```python
from build123d import *

# Parameters (mm, degrees)
BOSS_EXTRU_1_DEPTH = 8
CHANFREIN1_SIZE    = 3


with BuildPart() as part:
    # Esquisse1 → Boss.-Extru.1 (new body)
    with BuildSketch(Plane(origin=(0, 0, 0), x_dir=(1, 0, 0), z_dir=(0, 1, 0))):
        Polygon((0, 0), (0, 50.39696962), (9, 50.39696962), (50.39696962, 9), (50.39696962, 0), align=None)
    extrude(amount=BOSS_EXTRU_1_DEPTH)

    # Chanfrein1
    chanfrein1_edges = [part.edges().sort_by_distance(p)[0] for p in [
        (29.69848481, 8, -29.69848481),
        (4.5, 8, -50.39696962),
        (0, 8, -25.19848481),
        (25.19848481, 8, 0),
        (50.39696962, 8, -4.5),
    ]]
    chamfer(chanfrein1_edges, length=CHANFREIN1_SIZE)


solid = part.part
```
Work out the finished part from the listing and answer in its coordinate system (mm). Round coordinates to 2 decimals unless told otherwise and drop trailing zeros. Loops run counter-clockwise (first coordinate to the right, second up) from the corner with the lowest first, then second, coordinate; pieces in that order, holes last. Notation, with made-up numbers: (-2, 27) -> (15, 27) arc R26 cw to (15, 46) -> close; hole circle Ø9 at (10.5, 85.5). An arc over 180 degrees is marked (long way). Write each question's results on one line, items separated by ' | '. Start each with the question number.
1. Section B-B (z = -34) is taken. Determine the outline of the cut face in (x, y).
2. Given pin 1 Ø1.5 at (y, z) = (3, -24) entering from +X; pin 2 Ø1.5 at (x, y) = (17.5, 3) entering from -Z, each flat-ended and moving along its own axis, determine where each tip first touches the part or whether it passes through.
3. Section A-A (y = 3.25) is taken. Determine the outline of the cut face in (x, z), plus the area to 3 significant figures.
4. Section D-D (y = 6.75) is taken. Determine the outline of the cut face in (x, z), plus the area to 3 significant figures.
5. Find the intervals of material crossed by probe 1 along X at (y, z) = (6.5, -31); probe 2 along Z at (x, y) = (27, 3.25); probe 3 along X at (y, z) = (3.25, -31), in increasing order. Write a range as from..to.
6. Section C-C (x = 34.5) is taken. Determine the outline of the cut face in (y, z), plus the area to 3 significant figures.
Evaluation:
1) outline: (0, 0) -> (25.4, 0) -> (25.4, 5) -> (21.15, 8) -> (3, 8) -> (0, 5) -> close
2) pin 1: stops at x = 36.15 | pin 2: stops at z = -42.65
3) outline: (0, -50.4) -> (9, -50.4) -> (50.4, -9) -> (50.4, 0) -> (0, 0) -> close | area: 1,680 mm2
4) outline: (1.75, -48.65) -> (8.28, -48.65) -> (48.65, -8.28) -> (48.65, -1.75) -> (1.75, -1.75) -> close | area: 1,380 mm2
5) probe 1: x = 1.5..26.28 | probe 2: z = -32.4..0 | probe 3: x = 0..28.4
6) outline: (0, -24.9) -> (5, -24.9) -> (8, -20.65) -> (8, -3) -> (5, 0) -> (0, 0) -> close | area: 188 mm2
